from build123d import *

# Parameters (mm, degrees)
F0_W     = 94.4138541818
F0_H     = 118.8927069306
F1_DEPTH = 84.88416
F2_R     = 10.9607963201
F3_DEPTH = 12.7
F4_R     = 5.08
F5_T     = -2.54


# Not quite as in the source:
# - a shell that OpenCascade refuses in one call is made with other operations: the cavity is built on its own and cut out


with BuildPart() as f1:
    # F0 (on Top) → F1 (new body)
    with BuildSketch(Plane.XY):
        Rectangle(F0_W, F0_H)
    extrude(amount=F1_DEPTH)

    # F2 (on face) → F3 (join)
    with BuildSketch(Plane.XZ.offset(59.4463534653)):
        with Locations((0, 64.512334764)):
            Circle(F2_R)
    extrude(amount=F3_DEPTH)

    # F4
    f4_edges = [f1.edges().sort_by_distance(p)[0] for p in [
        (0, -59.446353, 84.88416),
        (47.206927, 0, 84.88416),
        (47.206927, 0, 0),
        (0, -59.446353, 0),
        (0, 59.446353, 84.88416),
        (-47.206927, 0, 84.88416),
        (0, 59.446353, 0),
        (47.206927, 59.446353, 42.44208),
        (47.206927, -59.446353, 42.44208),
        (-47.206927, 59.446353, 42.44208),
        (-47.206927, 0, 0),
        (-47.206927, -59.446353, 42.44208),
        (-10.960796, -72.146353, 64.512335),
    ]]
    fillet(f4_edges, radius=F4_R)

    # F5: a shell. OpenCascade refuses it in one call, so the cavity is built on its own and cut out:
    # the body offset inwards by the wall thickness, plus a prism from it out through each open face.
    f5_core = offset(f1.part, amount=F5_T, kind=Kind.INTERSECTION, mode=Mode.PRIVATE)
    f5_exits = [f5_core.faces().sort_by_distance(p)[0] for p in [
        (0, -69.606353, 64.512335),
    ]]
    add(f5_core, mode=Mode.SUBTRACT)
    extrude(f5_exits, amount=-F5_T, mode=Mode.SUBTRACT)


solid = f1.part
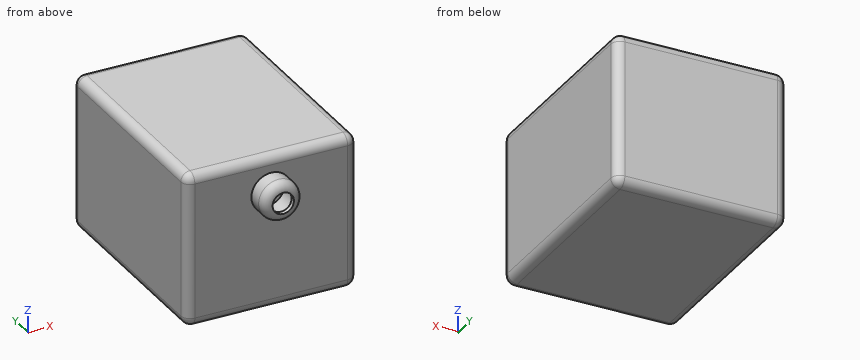
Part model, mm, in its own coordinate system. Round coordinates to 2 decimals unless told otherwise and drop trailing zeros. Write each loop counter-clockwise with the first axis right and the second up, starting at its lowest first coordinate (ties: lowest second). Pieces come first, ordered by that corner, then holes. Notation, with made-up numbers: (-1, -28.75) - (16, -28.75) arc R16 ccw to (16, -12.75) - close; hole circle Ø4 at (86.25, 84). An arc over 180 degrees is marked (long way). Use CSV: the item, a comma, the result in double quotes.
Item 1: Slice it at A-A, the plane z = 22.5. Write the cut outline in (x, y).
Results list:
outline,"(-47.21, -54.37) arc R5.08 ccw to (-42.13, -59.45) - (42.13, -59.45) arc R5.08 ccw to (47.21, -54.37) - (47.21, 54.37) arc R5.08 ccw to (42.13, 59.45) - (-42.13, 59.45) arc R5.08 ccw to (-47.21, 54.37) - close; hole (-44.67, -54.37) arc R2.54 ccw to (-42.13, -56.91) - (42.13, -56.91) arc R2.54 ccw to (44.67, -54.37) - (44.67, 54.37) arc R2.54 ccw to (42.13, 56.91) - (-42.13, 56.91) arc R2.54 ccw to (-44.67, 54.37) - close"
Item 2: Slice it at B-B, the plane y = 2.5. Write the cut outline in (x, z).
Results list:
outline,"(-47.21, 5.08) arc R5.08 ccw to (-42.13, 0) - (42.13, 0) arc R5.08 ccw to (47.21, 5.08) - (47.21, 79.8) arc R5.08 ccw to (42.13, 84.88) - (-42.13, 84.88) arc R5.08 ccw to (-47.21, 79.8) - close; hole (-44.67, 5.08) arc R2.54 ccw to (-42.13, 2.54) - (42.13, 2.54) arc R2.54 ccw to (44.67, 5.08) - (44.67, 79.8) arc R2.54 ccw to (42.13, 82.34) - (-42.13, 82.34) arc R2.54 ccw to (-44.67, 79.8) - close"
Item 3: Flat gauge pins, fed straight in: P1, Ø10.5, axis at x = 0, z = 64.51, coming from the -Y side; P2, Ø3, axis at x = -2.5, z = 16.5, coming from the -Y side. Where does each tip first touch, or does it go through?
Results list:
P1,"stops at y = 56.91"
P2,"stops at y = -59.45"
Item 4: Wall check: L1, parallel to X at y = 15, z = 40; L2, parallel to Y at x = -29, z = 67.5; L3, parallel to Z at x = 0, y = -61. Give the ranges that are in metal, low to high.
Results list:
L1,"x = -47.21 to -44.67, 44.67 to 47.21"
L2,"y = -59.45 to -56.91, 56.91 to 59.45"
L3,"z = 53.55 to 56.09, 72.93 to 75.47"
Item 5: Slice it at C-C, the plane x = 0. Write the cut outline in (y, z), then the cut area to 3 significant figures.
Results list:
outline,"(-72.15, 58.63) arc R5.08 ccw to (-67.07, 53.55) - (-59.45, 53.55) - (-59.45, 5.08) arc R5.08 ccw to (-54.37, 0) - (54.37, 0) arc R5.08 ccw to (59.45, 5.08) - (59.45, 79.8) arc R5.08 ccw to (54.37, 84.88) - (-54.37, 84.88) arc R5.08 ccw to (-59.45, 79.8) - (-59.45, 75.47) - (-67.07, 75.47) arc R5.08 ccw to (-72.15, 70.39) - (-69.61, 70.39) arc R2.54 cw to (-67.07, 72.93) - (-56.91, 72.93) - (-56.91, 79.8) arc R2.54 cw to (-54.37, 82.34) - (54.37, 82.34) arc R2.54 cw to (56.91, 79.8) - (56.91, 5.08) arc R2.54 cw to (54.37, 2.54) - (-54.37, 2.54) arc R2.54 cw to (-56.91, 5.08) - (-56.91, 56.09) - (-67.07, 56.09) arc R2.54 cw to (-69.61, 58.63) - close"
area,"1,020 mm²"
